from build123d import *

# Parameters (mm, degrees)
EXTRUDE_THIN1_DEPTH = 762
FILLET1_R           = 1.27


with BuildPart() as part:
    # Sketch1 → Extrude-Thin1 (new body)
    with BuildSketch(Plane.XY):
        with BuildLine():
            ThreePointArc((0, 4.7625), (-5.938970367, 0.015308043), (-11.1125, 5.586824141))
            Line((-11.1125, 5.586824141), (-11.1125, 7.9375))
            Line((-11.1125, 7.9375), (-12.7, 7.9375))
            ThreePointArc((-12.7, 7.9375), (-13.982491679, 16.639311629), (-17.720905139, 24.60113148))
            ThreePointArc((-17.720905139, 24.60113148), (-20.42299298, 29.566722219), (-22.225, 34.925))
            Line((-22.225, 34.925), (-24.60625, 34.925))
            Line((-24.60625, 34.925), (-24.60625, 52.3875))
            Line((-24.60625, 52.3875), (-27.78125, 52.3875))
            Line((-27.78125, 52.3875), (-27.78125, 76.2))
            Line((-27.78125, 76.2), (0, 76.2))
            Line((0, 76.2), (0, 69.85))
            Line((0, 69.85), (-1.27, 69.85))
            Line((-1.27, 69.85), (-1.27, 74.93))
            Line((-1.27, 74.93), (-26.51125, 74.93))
            Line((-26.51125, 74.93), (-26.51125, 53.6575))
            Line((-26.51125, 53.6575), (-23.33625, 53.6575))
            Line((-23.33625, 53.6575), (-23.33625, 36.195))
            Line((-23.33625, 36.195), (-21.209398438, 36.195))
            ThreePointArc((-21.209398438, 36.195), (-19.454378473, 30.532415703), (-16.662311672, 25.302758069))
            ThreePointArc((-16.662311672, 25.302758069), (-12.955869325, 17.611976621), (-11.455667045, 9.2075))
            Line((-11.455667045, 9.2075), (-9.8425, 9.2075))
            Line((-9.8425, 9.2075), (-9.8425, 5.586824141))
            ThreePointArc((-9.8425, 5.586824141), (-5.845020027, 1.28182821), (-1.256099738, 4.949885827))
            Line((-1.256099738, 4.949885827), (0, 4.7625))
        make_face()
    extrude(amount=-EXTRUDE_THIN1_DEPTH)

    # Fillet1
    fillet1_edges = [part.edges().sort_by_distance(p)[0] for p in [
        (-23.33625, 53.6575, -381),
        (-21.209398438, 36.195, -381),
        (-9.8425, 9.2075, -381),
        (-12.7, 7.9375, -381),
        (-24.60625, 34.925, -381),
        (-27.78125, 52.3875, -381),
        (-27.78125, 76.2, -381),
        (0, 76.2, -381),
    ]]
    fillet(fillet1_edges, radius=FILLET1_R)


solid = part.part
Could you check a few things on this model? Use its own coordinates, in mm. A direction names the side the tool comes from. Give positions to 0.01 mm unless a question says otherwise; leave off trailing zeros. Order: outer loops, then holes, each group sorted by start corner. A loop starts at its lowest first (then second) coordinate and runs counter-clockwise, first axis right, second up. Notation, with made-up numbers: (-32, -18) - (24, -18) arc R28 ccw to (24, 0) - close; hole circle Ø3 at (-29.75, 11). An arc over 180 degrees is marked (long way). One line per item, written item: value. Start each with the question number.
1. For faces 4 (the face through (-27.781, 64, -376)), 5 (the face through (-24.606, 44, -376)), 6 (the face through (-23.336, 44, -376)), 7 (the face through (-14, 74.93, -376)), which set-ups out of +Z, -Z, +X, -X, +Y, -Y let a thin tool reach every point of the face, with its end or its side?
2. If I drill on probe 1 along Y at (x, z) = (-6, -723); probe 2 along Y at (x, z) = (-22.5, -511) (3 decimals); probe 3 along X at (y, z) = (70.5, -681), over which ranges is the centre line in solid material (lowest first)?
3. Thinking about a two-plate mould opening in Y: for faces 1 (the face through (-12.993, 17.726, -375.666)), 2 (the face through (-14.13, 17.11, -375.67)), 3 (the face through (-24, 52, -762)), which applies, +Y half, -Y half, draft (parallel to the pull), parting line (faces both ways), or undercut?
4. Imagine slicing it at A-A on x = -5.5. List the corners of the cut face in (y, z) for me.
5. For P1, Ø1.5, axis at y = 44.5, z = -579.5, coming from the -X side; P2, Ø18, axis at y = 45, z = -555, coming from the -X side; P3, Ø2.5, axis at y = 6.5, z = -520, coming from the +X side; P4, Ø0.6, axis at x = -0.5, z = -278.5, coming from the -Y side, each with a flat end and sliding along its axis, tell me the tip position at first contact or that it passes through.
Values:
1. face 4: +Z, -Z, -X, +Y, -Y
1. face 5: +Z, -Z, -X, -Y
1. face 6: +Z, -Z, +X
1. face 7: +Z, -Z
2. probe 1: 0.02 to 1.3, 74.93 to 76.2
2. probe 2: 34.925 to 36.195, 74.93 to 76.2
2. probe 3: -27.78 to -26.51, -1.27 to 0
3. face 1: undercut
3. face 2: -Y half
3. face 3: draft
4. outline: (0, -762) - (1.27, -762) - (1.27, 0) - (0, 0) - close; (74.93, -762) - (76.2, -762) - (76.2, 0) - (74.93, 0) - close
5. P1: x = -24.61
5. P2: x = -27.78
5. P3: x = -9.83
5. P4: y = 2.61
